```python
from build123d import *

# Parameters (mm, degrees)
SKETCH_1_W               = 45
SKETCH_1_H               = 45
EXTRUDE_1_DEPTH          = 15.5
SKETCH_2_R               = 19.1
CUT_EXTRUDE_1_DEPTH      = 36.394208566
SKETCH_5_W               = 15
SKETCH_5_H               = 15.5
EXTRUDE_2_DEPTH          = 12
SKETCH_6_R               = 3
CUT_EXTRUDE_4_DEPTH      = 35
SKETCH_7_R               = 1.5
CUT_EXTRUDE_5_DEPTH      = 45.008522016
CUT_EXTRUDE_6_DEPTH      = 6
CUT_EXTRUDE_6_DEPTH_BACK = 6
SKETCH_9_R               = 4.25
CUT_EXTRUDE_7_DEPTH      = 12
CHAMFER_2_SIZE           = 1
CHAMFER_3_SIZE           = 1
CHAMFER_4_SIZE           = 1


# Some blends are built 0.0001 mm under size
with BuildPart() as part:
    # 草图1 → 凸台-拉伸1 (new body)
    with BuildSketch(Plane(origin=(0, 0, 0), x_dir=(1, 0, 0), z_dir=(0, 1, 0))):
        Rectangle(SKETCH_1_W, SKETCH_1_H)
    extrude(amount=EXTRUDE_1_DEPTH)

    # 草图2 → 切除-拉伸1 (cut, through all)
    with BuildSketch(Plane(origin=(0, 15.5, 0), x_dir=(1, 0, 0), z_dir=(0, 1, 0))):
        with Locations(Location((0, 0, 0), (0, 0, 270))):
            Circle(SKETCH_2_R)
    extrude(amount=-CUT_EXTRUDE_1_DEPTH, mode=Mode.SUBTRACT)

    # 草图5 → 凸台-拉伸2 (add)
    with BuildSketch(Plane(origin=(0, 0, -22.5), x_dir=(-1, 0, 0), z_dir=(0, 0, -1))):
        with Locations((14, 7.75)):
            Rectangle(SKETCH_5_W, SKETCH_5_H)
        with Locations((-14, 7.75)):
            Rectangle(SKETCH_5_W, SKETCH_5_H)
    extrude(amount=EXTRUDE_2_DEPTH)

    # 草图6 → 切除-拉伸4 (cut)
    with BuildSketch(Plane(origin=(0, 0, -34.5), x_dir=(-1, 0, 0), z_dir=(0, 0, -1))):
        with Locations((-14, 7.75)):
            Circle(SKETCH_6_R)
        with Locations((14, 7.75)):
            Circle(SKETCH_6_R)
    extrude(amount=-CUT_EXTRUDE_4_DEPTH, mode=Mode.SUBTRACT)

    # 草图7 → 切除-拉伸5 (cut, through all)
    with BuildSketch(Plane(origin=(0, 15.5, 0), x_dir=(1, 0, 0), z_dir=(0, 1, 0))):
        with Locations(Location((-19.5, 19.5, 0), (0, 0, 270))):
            Circle(SKETCH_7_R)
        with Locations(Location((19.5, 19.5, 0), (0, 0, 90))):
            Circle(SKETCH_7_R)
        with Locations(Location((19.5, -19.5, 0), (0, 0, 270))):
            Circle(SKETCH_7_R)
        with Locations(Location((-19.5, -19.5, 0), (0, 0, 90))):
            Circle(SKETCH_7_R)
    extrude(amount=-CUT_EXTRUDE_5_DEPTH, mode=Mode.SUBTRACT)

    # 草图8 → 切除-拉伸6 (cut, two sides: drawn at the far end of the back side and taken through both)
    with BuildSketch(Plane(origin=(0, 7.75, 0), x_dir=(-1, 0, 0), z_dir=(0, -1, 0)).offset(-CUT_EXTRUDE_6_DEPTH_BACK)):
        with BuildLine():
            Line((-8.874983497, 19.032463528), (-8.072008799, 17.310478732))
            ThreePointArc((-8.072008799, 17.310478732), (-15.1530488, 11.627343294), (-18.809828083, 3.316680193))
            Line((-18.809828083, 3.316680193), (-20.680962813, 3.646611731))
            ThreePointArc((-20.680962813, 3.646611731), (-16.660420146, 12.783990009), (-8.874983497, 19.032463528))
        make_face()
        with BuildLine():
            Line((20.680962813, 3.646611731), (18.809828083, 3.316680193))
            ThreePointArc((18.809828083, 3.316680193), (15.1530488, 11.627343294), (8.072008799, 17.310478732))
            Line((8.072008799, 17.310478732), (8.874983497, 19.032463528))
            ThreePointArc((8.874983497, 19.032463528), (16.660420146, 12.783990009), (20.680962813, 3.646611731))
        make_face()
    extrude(amount=CUT_EXTRUDE_6_DEPTH + CUT_EXTRUDE_6_DEPTH_BACK, mode=Mode.SUBTRACT)

    # 草图9 → 切除-拉伸7 (cut)
    with BuildSketch(Plane(origin=(0, 0, -34.5), x_dir=(-1, 0, 0), z_dir=(0, 0, -1))):
        with Locations((-14, 7.75)):
            Circle(SKETCH_9_R)
        with Locations((14, 7.75)):
            Circle(SKETCH_9_R)
    extrude(amount=-CUT_EXTRUDE_7_DEPTH, mode=Mode.SUBTRACT)

    # 倒角1
    # the kernel refuses this chamfer: 2 mm, written as the material it takes off along each edge
    with BuildSketch(Plane(origin=(-18.809828083, 1.75, -3.316680193), x_dir=(-0.09666023054018325, 0, 0.9953174367165073), z_dir=(0, 1, 0))) as chamfer_1_piece_1_section:
        with BuildLine():
            Line((1.811638226, -0.054831322), (-0.147910468, -1.899248595))
            Line((-0.147910468, -1.899248595), (0, 0))
            ThreePointArc((0, 0), (0.933514183, -0.049753736), (1.811638226, -0.054831322))
        make_face()
    chamfer_1_piece_1 = extrude(amount=12, mode=Mode.PRIVATE)
    chamfer_1_piece_1 = chamfer_1_piece_1 & Plane(origin=(0, 7.75, 0), x_dir=(-0.42261826174070266, 0, -0.9063077870366485), z_dir=(0, 1, 0)) * Cylinder(21, 32, mode=Mode.PRIVATE)
    add(chamfer_1_piece_1, mode=Mode.SUBTRACT)
    with BuildSketch(Plane(origin=(18.809828083, 13.75, -3.316680193), x_dir=(0.09666023054018283, 0, 0.9953174367165073), z_dir=(0, -1, 0))) as chamfer_1_piece_2_section:
        with BuildLine():
            Line((1.811638226, -0.054831322), (-0.147910468, -1.899248595))
            Line((-0.147910468, -1.899248595), (0, 0))
            ThreePointArc((0, 0), (0.933514183, -0.049753736), (1.811638226, -0.054831322))
        make_face()
    chamfer_1_piece_2 = extrude(amount=12, mode=Mode.PRIVATE)
    chamfer_1_piece_2 = chamfer_1_piece_2 & Plane(origin=(0, 7.75, 0), x_dir=(0.9848077530122075, 0, -0.17364817766693397), z_dir=(0, 1, 0)) * Cylinder(21, 32, mode=Mode.PRIVATE)
    add(chamfer_1_piece_2, mode=Mode.SUBTRACT)

    # 倒角2
    chamfer_2_edges = [part.edges().sort_by_distance(p)[0] for p in [
        (22.5, 7.75, 22.5),
        (-22.5, 7.75, 22.5),
        (-22.5, 7.75, -22.5),
        (22.5, 7.75, -22.5),
    ]]
    chamfer(chamfer_2_edges, length=CHAMFER_2_SIZE - 0.0001)  # a hair under: the kernel refuses the full size

    # 倒角3
    chamfer_3_edges = [part.edges().sort_by_distance(p)[0] for p in [
        (18.25, 7.75, -22.5),
        (-9.75, 7.75, -22.5),
    ]]
    chamfer(chamfer_3_edges, length=CHAMFER_3_SIZE)

    # 倒角4
    chamfer_4_edges = [part.edges().sort_by_distance(p)[0] for p in [
        (6.5, 7.75, -34.5),
        (14, 15.5, -34.5),
        (21.5, 7.75, -34.5),
        (14, 0, -34.5),
        (-21.5, 7.75, -34.5),
        (-14, 15.5, -34.5),
        (-6.5, 7.75, -34.5),
        (-14, 0, -34.5),
    ]]
    chamfer(chamfer_4_edges, length=CHAMFER_4_SIZE)


solid = part.part
```
Can you work these out from the model? Positions are in its coordinate system, mm. A direction names the side the tool comes from. Give positions to 0.01 mm unless a question says otherwise; leave off trailing zeros. Write each loop counter-clockwise with the first axis right and the second up, starting at its lowest first coordinate (ties: lowest second). Pieces come first, ordered by that corner, then holes. Notation, with made-up numbers: (80.25, 31) -> (119.25, 31) arc R11 ccw to (119.25, 36) -> close; hole circle Ø6 at (23, 46). An arc over 180 degrees is marked (long way). Write item = value, one per line.
(1) Suppose I cut it at A-A on z = -29. Write out the boundary of the cut face in (x, y).
Worked out:
outline = (-21.5, 0) -> (-6.5, 0) -> (-6.5, 15.5) -> (-21.5, 15.5) -> close; (6.5, 0) -> (21.5, 0) -> (21.5, 15.5) -> (6.5, 15.5) -> close; hole circle Ø8.5 at (-14, 7.75); hole circle Ø8.5 at (14, 7.75)
(2) Suppose I cut it at B-B on x = -14. Write out the boundary of the cut face in (y, z), then the cut area to 3 significant figures.
Worked out:
outline = (0, -33.5) -> (1, -34.5) -> (3.5, -34.5) -> (3.5, -23.5) -> (4.5, -22.5) -> (4.75, -22.5) -> (4.75, -15.65) -> (1.75, -15.65) -> (1.75, -12.99) -> (0, -12.99) -> close; (0, 12.99) -> (15.5, 12.99) -> (15.5, 22.5) -> (0, 22.5) -> close; (10.75, -22.5) -> (11, -22.5) -> (12, -23.5) -> (12, -34.5) -> (14.5, -34.5) -> (15.5, -33.5) -> (15.5, -12.99) -> (13.75, -12.99) -> (13.75, -15.65) -> (10.75, -15.65) -> close
area = 306 mm^2
(3) I need wall thicknesses on probe 1 along X at (y, z) = (7.25, 19.5); probe 2 along X at (y, z) = (7.75, -17); probe 3 along Y at (x, z) = (14, -28.5). Which ranges of each line are inside material? Lowest first, please. Write a range as from..to.
Worked out:
probe_1 = -22.5..-21, -18..18, 21..22.5
probe_2 = -22.5..-17, 17..22.5
probe_3 = 0..3.5, 12..15.5
(4) Suppose I cut it at D-D on x = -3.5. Write out the boundary of the cut face in (y, z), then the cut area to 3 significant figures.
Worked out:
outline = (0, -22.5) -> (15.5, -22.5) -> (15.5, -18.78) -> (0, -18.78) -> close; (0, 18.78) -> (15.5, 18.78) -> (15.5, 22.5) -> (0, 22.5) -> close
area = 115 mm^2
(5) I'm going to push flat-ended pins straight in: P1, Ø3.5, axis at y = 7, z = -30, coming from the +X side; P2, Ø7, axis at x = -14.5, y = 8, coming from the -Z side; P3, Ø5, axis at x = 14, y = 7.75, coming from the -Z side. Where does each tip first touch, or does it pass through?
Worked out:
P1 = 21.5
P2 = -23.31
P3 = 9.62
(6) Thinking about a two-plate mould opening in Z: for faces 5 (the face through (0, 8, -22.5)), 6 (the face through (8.479, 7.834, -18.184)), 7 (the face through (12, 4, -29)), which applies, released by +Z, released by -Z, zero draft, split by the parting line, or undercut?
Worked out:
face_5 = released by -Z
face_6 = undercut
face_7 = zero draft
(7) For faces 1 (the face through (21.5, 8, -28)), 2 (the face through (-16, 4, -29)), 3 (the face through (16, 1.75, -11)), 4 (the face through (-11, 11, -34.5)), which set-ups out of +Z, -Z, +X, -X, +Y, -Y let a thin tool reach every point of the face, with its end or its side?
Worked out:
face_1 = -Z, +X, +Y, -Y
face_2 = -Z
face_3 = none
face_4 = -Z, +X, -X, +Y, -Y
(8) Suppose I cut it at C-C on z = 0. Write out the boundary of the cut face in (x, y).
Worked out:
outline = (-22.5, 0) -> (-19.1, 0) -> (-19.1, 15.5) -> (-22.5, 15.5) -> close; (19.1, 0) -> (22.5, 0) -> (22.5, 15.5) -> (19.1, 15.5) -> close
